```python
from build123d import *

# Parameters (mm, degrees)
BOSS_EXTRUDE1_DEPTH      = 25.4
BOSS_EXTRUDE1_DEPTH_BACK = 34.925
CUT_EXTRUDE4_DEPTH       = 63.941922635
CUT_EXTRUDE5_DEPTH       = 46.01339384
SKETCH14_R               = 3.2893
CUT_EXTRUDE6_DEPTH       = 46.01339384
CUT_EXTRUDE7_DEPTH       = 12.7
CUT_EXTRUDE7_DEPTH_BACK  = 38.1
SKETCH15_R               = 12.7


with BuildPart() as part:
    # Sketch1 → Boss-Extrude1 (new, two sides: drawn at the far end of the back side and taken through both)
    with BuildSketch(Plane(origin=(0, 0, 0), x_dir=(0, 0, -1), z_dir=(1, 0, 0)).offset(-BOSS_EXTRUDE1_DEPTH_BACK)):
        with BuildLine():
            Line((-10.16, 12.7), (10.16, 12.7))
            ThreePointArc((10.16, 12.7), (11.956051224, 11.956051224), (12.7, 10.16))
            Line((12.7, 10.16), (12.7, -10.16))
            ThreePointArc((12.7, -10.16), (11.956051224, -11.956051224), (10.16, -12.7))
            Line((10.16, -12.7), (-10.16, -12.7))
            ThreePointArc((-10.16, -12.7), (-11.956051224, -11.956051224), (-12.7, -10.16))
            Line((-12.7, -10.16), (-12.7, 10.16))
            ThreePointArc((-12.7, 10.16), (-11.956051224, 11.956051224), (-10.16, 12.7))
        make_face()
    extrude(amount=BOSS_EXTRUDE1_DEPTH + BOSS_EXTRUDE1_DEPTH_BACK)

    # Sketch11 → Cut-Extrude4 (cut, through all)
    with BuildSketch(Plane(origin=(25.4, 0, 0), x_dir=(0, 0, -1), z_dir=(1, 0, 0))):
        with BuildLine():
            Line((-10.6045, 11.1125), (10.6045, 11.1125))
            ThreePointArc((10.6045, 11.1125), (10.963710245, 10.963710245), (11.1125, 10.6045))
            Line((11.1125, 10.6045), (11.1125, -10.6045))
            ThreePointArc((11.1125, -10.6045), (10.963710245, -10.963710245), (10.6045, -11.1125))
            Line((10.6045, -11.1125), (-10.6045, -11.1125))
            ThreePointArc((-10.6045, -11.1125), (-10.963710245, -10.963710245), (-11.1125, -10.6045))
            Line((-11.1125, -10.6045), (-11.1125, 10.6045))
            ThreePointArc((-11.1125, 10.6045), (-10.963710245, 10.963710245), (-10.6045, 11.1125))
        make_face()
    extrude(amount=-CUT_EXTRUDE4_DEPTH, mode=Mode.SUBTRACT)

    # Sketch12 → Cut-Extrude5 (cut, through all)
    with BuildSketch(Plane(origin=(0, 12.7, 0), x_dir=(1, 0, 0), z_dir=(0, 1, 0))):
        with BuildLine():
            Line((0, 12.7), (50.8, 12.7))
            Line((50.8, 12.7), (50.8, -12.7))
            Line((50.8, -12.7), (0, -12.7))
            Line((0, -12.7), (19.444424463, -7.686083637))
            ThreePointArc((19.444424463, -7.686083637), (25.4, 0), (19.444424463, 7.686083637))
            Line((19.444424463, 7.686083637), (0, 12.7))
        make_face()
    extrude(amount=-CUT_EXTRUDE5_DEPTH, mode=Mode.SUBTRACT)

    # Sketch14 → Cut-Extrude6 (cut, through all)
    with BuildSketch(Plane(origin=(0, 12.7, 0), x_dir=(1, 0, 0), z_dir=(0, 1, 0))):
        with Locations(Location((17.4625, 0, 0), (0, 0, 270))):
            Circle(SKETCH14_R)
    extrude(amount=-CUT_EXTRUDE6_DEPTH, mode=Mode.SUBTRACT)

    # Sketch15 → Cut-Extrude7 (cut, two sides: drawn at the far end of the back side and taken through both)
    with BuildSketch(Plane(origin=(-28.000601556, -14.856223036, 12.7), x_dir=(0.9956294808615993, 0.00690045849591187, 0.09313603229582208), z_dir=(-0.09339131029845452, 0.0735646591533628, 0.9929080038374085)).offset(-CUT_EXTRUDE7_DEPTH_BACK)):
        Circle(SKETCH15_R)
    extrude(amount=CUT_EXTRUDE7_DEPTH + CUT_EXTRUDE7_DEPTH_BACK, mode=Mode.SUBTRACT)


solid = part.part
```
Work out the finished part from the listing and answer in its coordinate system (mm). A direction names the side the tool comes from. Round coordinates to 2 decimals unless told otherwise and drop trailing zeros. Loops run counter-clockwise (first coordinate to the right, second up) from the corner with the lowest first, then second, coordinate; pieces in that order, holes last.
(1) This flat-tipped pin is pushed along its axis until it touches: P1, Ø12, axis at y = -7.5, z = -5.5, coming from the +X side. Where does it stop, or does it pass through?
Computed values:
P1: stops at x = 25.37
(2) The part is cut by section D-D, the plane y = -3. Give the number of separate pieces and of enclosed holes in the cut face, and give its area (3 significant figures).
Computed values:
separate pieces: 3
enclosed holes: 0
area: 106 mm2
(3) The part is cut by section B-B, the plane y = 5.75. Give the vertices of the cut face in (x, z) (1 decimal).
Computed values:
outline: (-34.9, -12.7) - (0, -12.7) - (6.2, -11.1) - (-34.9, -11.1) - close; (-34.9, 11.1) - (6.2, 11.1) - (0, 12.7) - (-34.9, 12.7) - close
(4) Find the intervals of material crossed by L1, parallel to Y at x = 8.5, z = 4.75; L2, parallel to X at y = -11.8, z = 0, in increasing order.
Computed values:
L1: y = -12.7 to -11.11, 11.11 to 12.7
L2: x = -14.72 to 14.17, 20.75 to 25.4
(5) The mould has two halves that part along X. Classify faces 3 (the cylindrical face through (25.4, -11.9, 0.1)), 4 (the flat face through (-5, 12.7, 0)), 5 (the cylindrical face through (14.544, 11.917, 1.518)), 6 (the cylindrical face through (-14.77, -11.92, 1.23)): pulls with the +X half, pulls with the -X half, needs draft (parallel to the pull), parting line crosses it, or undercut.
Computed values:
face 3: pulls with the +X half
face 4: needs draft
face 5: undercut
face 6: undercut
(6) For faces 1 (the cylindrical face through (-17.826, 11.936, 11.976)), 2 (the flat face through (-4, 11.112, 0)), determine the directions among +Z, -Z, +X, -X, +Y, -Y from which every point of the face is accessible in a straight line to the end or side of a thin tool.
Computed values:
face 1: +Z, +X, -X, +Y
face 2: +X, -X
(7) The part is cut by section A-A, the plane x = 11. Give the vertices of the cut face in (y, z), and give its area (3 significant figures).
Computed values:
outline: (-12.7, -9.86) - (-11.11, -9.86) - (-11.11, 9.86) - (-12.7, 9.86) - close; (11.11, -9.86) - (12.7, -9.86) - (12.7, 9.86) - (11.11, 9.86) - close
area: 62.6 mm2
(8) The part is cut by section C-C, the plane x = 3. Give the vertices of the cut face in (y, z), and give its area (3 significant figures).
Computed values:
outline: (-12.7, -10.16) arc R2.54 ccw to (-11.99, -11.93) - (11.99, -11.93) arc R2.54 ccw to (12.7, -10.16) - (12.7, 10.16) arc R2.54 ccw to (11.99, 11.93) - (-11.99, 11.93) arc R2.54 ccw to (-12.7, 10.16) - close; hole (-11.11, -10.6) arc R0.51 ccw to (-10.6, -11.11) - (10.6, -11.11) arc R0.51 ccw to (11.11, -10.6) - (11.11, 10.6) arc R0.51 ccw to (10.6, 11.11) - (-10.6, 11.11) arc R0.51 ccw to (-11.11, 10.6) - close
area: 111 mm2
